Drawing for the job (mm, zero at the part's lowest x, y, z). A direction names the side the tool comes from. Round coordinates to 2 decimals unless told otherwise and drop trailing zeros. Write each loop counter-clockwise with the first axis right and the second up, starting at its lowest first coordinate (ties: lowest second). Pieces come first, ordered by that corner, then holes. Notation, with made-up numbers: (-29.5, 10) -> (1.5, 10) arc R11 cw to (1.5, 19) -> close; hole circle Ø11 at (-35.5, -12). An arc over 180 degrees is marked (long way). Answer in a Markdown table with one row per item. Add a question column.
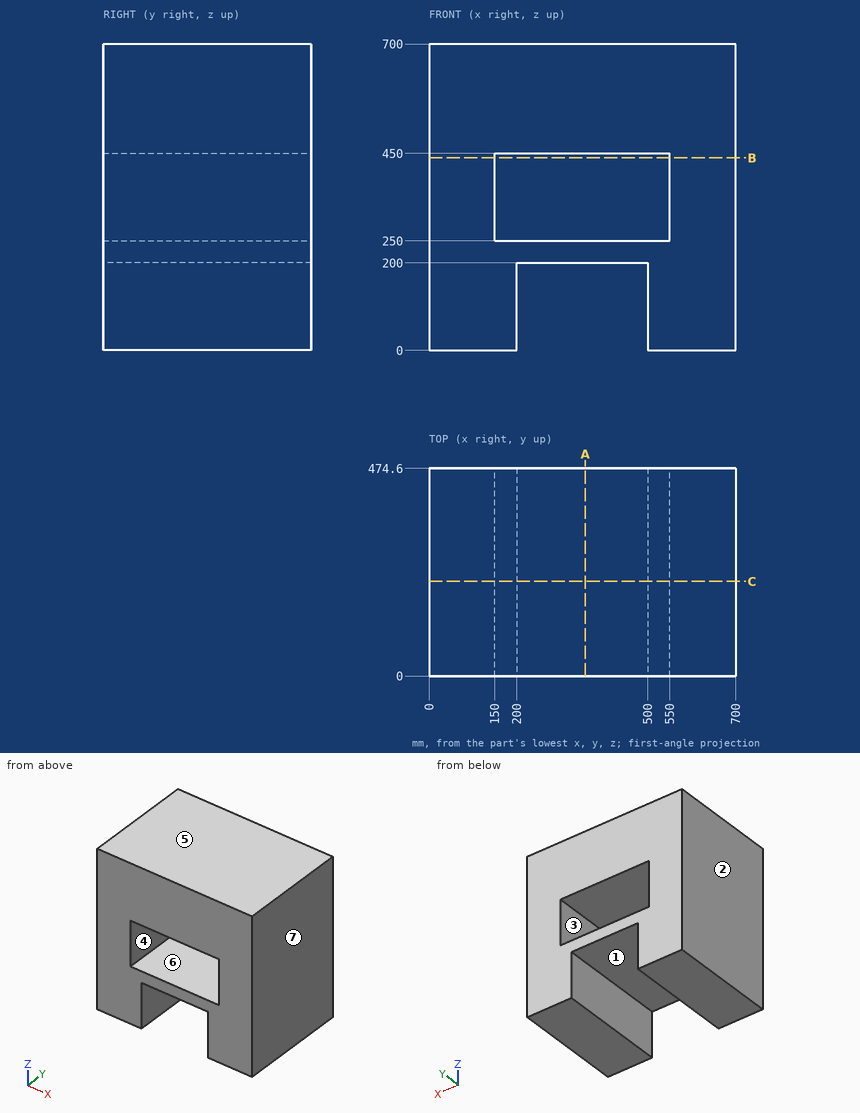
(1) Saw through at A-A (x = 357). List the corners of the cut face in (y, z).
(2) Saw through at B-B (z = 440). List the corners of the cut face in (x, y), plus the area to 3 significant figures.
(3) Probe line 1 along Z through (x, y) = (519.5, 373.5); line 2 along Z through (x, y) = (393, 342.5); line 3 along X through (y, z) = (271, 359.5). List the from-to ranges inside material, lowest first.
(4) Saw through at C-C (y = 216.5). List the corners of the cut face in (x, z), plus the area to 3 significant figures.
(5) Which spindle directions (+Z, -Z, +X, -X, +Y, -Y) get a long thin tool onto all of the face, cutting with end or side? Do the marked faces 1, 2 and 3. Say none if no direction does.
(6) Mould opens along X. For the marked faces 4, 5, 6 and 7 say: pulls with the +X half, pulls with the -X half, needs draft (parallel to the pull), parting line crosses it, or undercut.
Answer sheet:
| question | item | result |
|---|---|---|
| 1 | outline | (0, 200) -> (474.6, 200) -> (474.6, 250) -> (0, 250) -> close; (0, 450) -> (474.6, 450) -> (474.6, 700) -> (0, 700) -> close |
| 2 | outline | (0, 0) -> (150, 0) -> (150, 474.6) -> (0, 474.6) -> close; (550, 0) -> (700, 0) -> (700, 474.6) -> (550, 474.6) -> close |
| 2 | area | 142,000 mm² |
| 3 | line 1 | z = 0 to 250, 450 to 700 |
| 3 | line 2 | z = 200 to 250, 450 to 700 |
| 3 | line 3 | x = 0 to 150, 550 to 700 |
| 4 | outline | (0, 0) -> (200, 0) -> (200, 200) -> (500, 200) -> (500, 0) -> (700, 0) -> (700, 700) -> (0, 700) -> close; hole (150, 250) -> (550, 250) -> (550, 450) -> (150, 450) -> close |
| 4 | area | 350,000 mm² |
| 5 | face 1 | -Z, +Y, -Y |
| 5 | face 2 | +Z, -Z, -X, +Y, -Y |
| 5 | face 3 | +Y, -Y |
| 6 | face 4 | undercut |
| 6 | face 5 | needs draft |
| 6 | face 6 | undercut |
| 6 | face 7 | pulls with the +X half |
